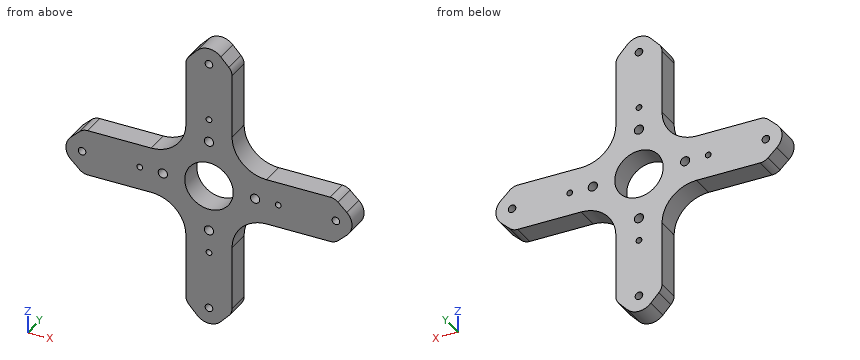
```python
from build123d import *

# Parameters (mm, degrees)
SKETCH1_R             = 2
SKETCH1_R_2           = 10.5
BOSS_EXTRUDE1_DEPTH   = 10
FILLET1_R             = 15
FILLET2_R             = 5
M4X0_7_TAPPED_HOLE1_D = 3.3
M3X0_5_TAPPED_HOLE1_D = 2.5


with BuildPart() as part:
    # Sketch1 → Boss-Extrude1 (new body)
    with BuildSketch(Plane(origin=(0, 0, 0), x_dir=(1, 0, 0), z_dir=(0, 1, 0))):
        with BuildLine():
            Line((10, 10), (54.556312231, 10))
            Line((54.556312231, 10), (59.781818182, 5.112163424))
            ThreePointArc((59.781818182, 5.112163424), (62, 0), (59.781818182, -5.112163424))
            Line((59.781818182, -5.112163424), (54.556312231, -10))
            Line((54.556312231, -10), (10, -10))
            Line((10, -10), (10, -54.556312231))
            Line((10, -54.556312231), (5.112163424, -59.781818182))
            ThreePointArc((5.112163424, -59.781818182), (0, -62), (-5.112163424, -59.781818182))
            Line((-5.112163424, -59.781818182), (-10, -54.556312231))
            Line((-10, -54.556312231), (-10, -10))
            Line((-10, -10), (-54.556312231, -10))
            Line((-54.556312231, -10), (-59.781818182, -5.112163424))
            ThreePointArc((-59.781818182, -5.112163424), (-62, 0), (-59.781818182, 5.112163424))
            Line((-59.781818182, 5.112163424), (-54.556312231, 10))
            Line((-54.556312231, 10), (-10, 10))
            Line((-10, 10), (-10, 54.556312231))
            Line((-10, 54.556312231), (-5.112163424, 59.781818182))
            ThreePointArc((-5.112163424, 59.781818182), (0, 62), (5.112163424, 59.781818182))
            Line((5.112163424, 59.781818182), (10, 54.556312231))
            Line((10, 54.556312231), (10, 10))
        make_face()
        with Locations(Location((-20, 0, 0), (0, 0, 270))):
            Circle(SKETCH1_R, mode=Mode.SUBTRACT)
        with Locations(Location((0, 20, 0), (0, 0, 270))):
            Circle(SKETCH1_R, mode=Mode.SUBTRACT)
        with Locations(Location((20, 0, 0), (0, 0, 270))):
            Circle(SKETCH1_R, mode=Mode.SUBTRACT)
        with Locations(Location((0, -20, 0), (0, 0, 270))):
            Circle(SKETCH1_R, mode=Mode.SUBTRACT)
        with Locations(Location((0, 0, 0), (0, 0, 270))):
            Circle(SKETCH1_R_2, mode=Mode.SUBTRACT)
    extrude(amount=BOSS_EXTRUDE1_DEPTH)

    # Fillet1
    fillet1_edges = [part.edges().sort_by_distance(p)[0] for p in [
        (10, 5, -10),
        (10, 5, 10),
        (-10, 5, 10),
        (-10, 5, -10),
    ]]
    fillet(fillet1_edges, radius=FILLET1_R)

    # Fillet2
    fillet2_edges = [part.edges().sort_by_distance(p)[0] for p in [
        (54.556312231, 5, -10),
        (54.556312231, 5, 10),
        (10, 5, 54.556312231),
        (-10, 5, 54.556312231),
        (-54.556312231, 5, 10),
        (-54.556312231, 5, -10),
        (-10, 5, -54.556312231),
        (10, 5, -54.556312231),
    ]]
    fillet(fillet2_edges, radius=FILLET2_R)

    # M4x0.7 Tapped Hole1 (through all)
    with Locations(Plane(origin=(0, 0, 0), x_dir=(-1, 0, 0), z_dir=(0, -1, 0))):
        with Locations((0, -55), (-55, 0), (0, 55), (55, 0)):
            Hole(M4X0_7_TAPPED_HOLE1_D / 2)

    # M3x0.5 Tapped Hole1 (through all)
    with Locations(Plane(origin=(0, 0, 0), x_dir=(-1, 0, 0), z_dir=(0, -1, 0))):
        with Locations((0, -30), (-30, 0), (0, 30), (30, 0), (0, 0)):
            Hole(M3X0_5_TAPPED_HOLE1_D / 2)


solid = part.part
```
The listing builds one solid part. Answer for the finished solid, in the listing's coordinates (mm). Coordinates: 2 decimals unless noted, no trailing zeros. Loops run counter-clockwise (first coordinate to the right, second up) from the corner with the lowest first, then second, coordinate; pieces in that order, holes last. Notation, with made-up numbers: (7, 29) -> (60, 29) arc R31 cw to (60, 66) -> close; hole circle Ø3 at (53, 32.25). An arc over 180 degrees is marked (long way). Return JSON: item names as keys, results as strings. Group by question number.
(1) A cutting plane is placed at A-A on x = -20. Write down the section's boundary in (y, z).
(2) A cutting plane is placed at C-C on y = 4.25. Count the separate pieces of the cut face and the enclosed holes in it, and give its area (3 significant figures).
(3) A cutting plane is placed at D-D on x = 36. Write down the section's boundary in (y, z), and give its area (3 significant figures).
(4) Find the intervals of material crossed by probe 1 along X at (y, z) = (4, 39); probe 2 along Z at (x, y) = (-21, 6.25), in increasing order. Write a range as from..to.
(5) Given pin 1 Ø3 at (y, z) = (8, 7.5) entering from +X; pin 2 Ø5 at (y, z) = (4.5, -37.5) entering from +X; pin 3 Ø1 at (y, z) = (4.5, 10) entering from -X, each flat-ended and moving along its own axis, determine where each tip first touches the part or whether it passes through.
(6) A cutting plane is placed at B-B on z = -20. Write down the section's boundary in (x, y), and give its area (3 significant figures).
The answers:
{
 "1": {"outline": "(0, -10.86) -> (10, -10.86) -> (10, -2) -> (0, -2) -> close; (0, 2) -> (10, 2) -> (10, 10.86) -> (0, 10.86) -> close"},
 "2": {"separate pieces": "1", "enclosed holes": "13", "area": "4,080 mm^2"},
 "3": {"outline": "(0, -10) -> (10, -10) -> (10, 10) -> (0, 10) -> close", "area": "200 mm^2"},
 "4": {"probe 1": "x = -10..10", "probe 2": "z = -10.54..-1.73, 1.73..10.54"},
 "5": {"pin 1": "stops at x = 58.83", "pin 2": "stops at x = 10", "pin 3": "stops at x = -54.76"},
 "6": {"outline": "(-10.86, 0) -> (-2, 0) -> (-2, 10) -> (-10.86, 10) -> close; (2, 0) -> (10.86, 0) -> (10.86, 10) -> (2, 10) -> close", "area": "177 mm^2"}
}
